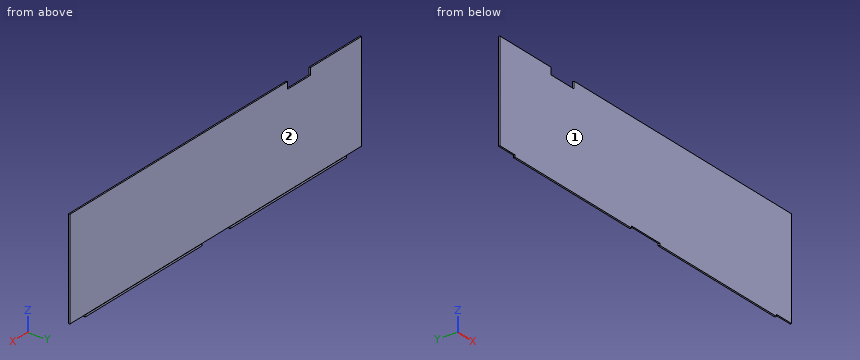
```python
from build123d import *

# Parameters (mm, degrees)
SKETCH1_W           = 635.3556
SKETCH1_H           = 165.1
BOSS_EXTRUDE1_DEPTH = 1.143
SKETCH2_W           = 254
SKETCH2_H           = 2.7305
BOSS_EXTRUDE2_DEPTH = 3.175
SKETCH3_W           = 50.8
SKETCH3_H           = 11.194977228
SKETCH3_H_2         = 11.572519195
CUT_EXTRUDE1_DEPTH  = 330.052299594


with BuildPart() as part:
    # Sketch1 → Boss-Extrude1 (new, symmetric)
    with BuildSketch(Plane(origin=(0, 0, 0), x_dir=(1, 0, 0), z_dir=(0, 1, 0))):
        Rectangle(SKETCH1_W, SKETCH1_H)
    extrude(amount=BOSS_EXTRUDE1_DEPTH, both=True)

    # Sketch2 → Boss-Extrude2 (add)
    with BuildSketch(Plane(origin=(0, 0, -82.55), x_dir=(-1, 0, 0), z_dir=(0, 0, -1))):
        with Locations((-157.8229, 0.22225)):
            Rectangle(SKETCH2_W, SKETCH2_H)
        with Locations((157.8229, 0.22225)):
            Rectangle(SKETCH2_W, SKETCH2_H)
    extrude(amount=BOSS_EXTRUDE2_DEPTH)

    # Sketch3 → Cut-Extrude1 (cut, through all)
    with BuildSketch(Plane.XZ.offset(1.143)):
        with Locations((-181.370930865, 88.147488614)):
            Rectangle(SKETCH3_W, SKETCH3_H)
        with Locations((-181.370930865, 76.763740403)):
            Rectangle(SKETCH3_W, SKETCH3_H_2)
    extrude(amount=-CUT_EXTRUDE1_DEPTH, mode=Mode.SUBTRACT)


solid = part.part
```
Could you check a few things on this model? Use its own coordinates, in mm. Face numbers are marked on the shaded views. A direction names the side the tool comes from. Round coordinates to 2 decimals unless told otherwise and drop trailing zeros. Loops run counter-clockwise (first coordinate to the right, second up) from the corner with the lowest first, then second, coordinate; pieces in that order, holes last.
Q1. Please list where these lines run through material, in increasing order: L1, parallel to X at y = 0, z = 75; L2, parallel to Y at x = 116, z = 43; L3, parallel to Z at x = -127, y = 1.3 (3 decimals).
Q2. I want a section at B-B (z = -69.5). Write out the boundary of the cut face in (x, y), and give its area (3 significant figures).
Q3. On a 3-axis mill with a long thin cutter (end or side, diameter ignored), from which of +Z, -Z, +X, -X, +Y, -Y can I reach the whole of each face in a straight line? I mean the marked faces 1 and 2. Say none if no direction works.
Q4. For P1, Ø6, axis at x = 28, z = -2.5, coming from the +Y side; P2, Ø0.8, axis at y = 0.5, z = -84.5, coming from the -X side; P3, Ø1.4, axis at y = 0.5, z = -84, coming from the +X side, each with a flat end and sliding along its axis, tell me the tip position at first contact or that it passes through.
Answer below:
1. L1: x = -317.68 to -206.77, -155.97 to 317.68
1. L2: y = -1.14 to 1.14
1. L3: z = -85.725 to -82.55
2. outline: (-317.68, -1.14) - (317.68, -1.14) - (317.68, 1.14) - (-317.68, 1.14) - close
2. area: 1,450 mm2
3. face 1: +Z, -Z, +X, -X, -Y
3. face 2: +Z, +X, -X, +Y
4. P1: stops at y = 1.14
4. P2: stops at x = -284.82
4. P3: stops at x = 284.82
